from build123d import *

# Parameters (mm, degrees)
F0_R     = 6.35
F1_DEPTH = 3.81
F2_R     = 2.54
F3_DEPTH = 5.08
F6_D     = 3.175
F6_DEPTH = 2.032
F6_TIP   = 0.9538662327
F7_D     = 3.175
F7_DEPTH = 2.032
F7_TIP   = 0.9538662327


with BuildPart() as f1:
    # F0 (on Top) → F1 (new body)
    with BuildSketch(Plane.XY):
        Circle(F0_R)
    extrude(amount=F1_DEPTH)

    # F2 (on face) → F3 (join)
    with BuildSketch(Plane.XY.offset(3.81)):
        Circle(F2_R)
    extrude(amount=F3_DEPTH)

    # F6
    with Locations(Plane.XY.offset(3.81)):
        with Locations((-4.445, 0)):
            Hole(F6_D / 2, depth=F6_DEPTH)
            with Locations((0, 0, -(F6_DEPTH + F6_TIP / 2))):  # 118° drill point
                Cone(0, F6_D / 2, F6_TIP, mode=Mode.SUBTRACT)

    # F7
    with Locations(Plane.XY.offset(3.81)):
        with Locations((4.445, 0)):
            Hole(F7_D / 2, depth=F7_DEPTH)
            with Locations((0, 0, -(F7_DEPTH + F7_TIP / 2))):  # 118° drill point
                Cone(0, F7_D / 2, F7_TIP, mode=Mode.SUBTRACT)


solid = f1.part
Verification items for the finished model (mm, model axes). A direction names the side the tool comes from. Coordinates: 2 decimals unless noted, no trailing zeros. Order: outer loops, then holes, each group sorted by start corner. A loop starts at its lowest first (then second) coordinate and runs counter-clockwise, first axis right, second up.
Item 1: Section check B-B, the plane z = 4.5. Enter the section's corners in (x, y), then the cut area to 3 significant figures.
Filled in:
outline: circle Ø5.08 at (0, 0)
area: 20.3 mm2
Item 2: Release check for a two-part mould opening along Y. For faces 1 (the face through (-1.38, -6.2, 1.88)), 2 (the face through (0, 0, 0)), 3 (the face through (-4.18, 0.08, 0.99)) record: +Y half, -Y half, draft (parallel to the pull), parting line (faces both ways), or undercut.
Filled in:
face 1: parting line
face 2: draft
face 3: undercut
Item 3: Section check D-D, the plane y = -4.25. Enter the section's corners in (x, z), then the cut area to 3 significant figures.
Filled in:
outline: (-4.72, 0) - (4.72, 0) - (4.72, 3.81) - (-4.72, 3.81) - close
area: 36.0 mm2
Item 4: Access from +Z, -Z, +X, -X, +Y, -Y to the whole of each face (thin tool, end or side, straight path). Record for faces 4 (the face through (6.03, 0.07, 2.78)), 5 (the face through (0, 0, 8.89)).
Filled in:
face 4: +Z
face 5: +Z, +X, -X, +Y, -Y
Item 5: Material ranges on L1, parallel to X at y = 1, z = 3.5; L2, parallel to Z at x = -3.75, y = -1.5; L3, parallel to Y at x = 0, z = 4.75, recorded low to high.
Filled in:
L1: x = -6.27 to -5.68, -3.21 to 3.21, 5.68 to 6.27
L2: z = 0 to 3.81
L3: y = -2.54 to 2.54
Item 6: Section check A-A, the plane x = 0. Enter the section's corners in (y, z).
Filled in:
outline: (-6.35, 0) - (6.35, 0) - (6.35, 3.81) - (2.54, 3.81) - (2.54, 8.89) - (-2.54, 8.89) - (-2.54, 3.81) - (-6.35, 3.81) - close
Item 7: Depth check by flat-ended pin: pin 1 (3 mm diameter, centred on y = 2, z = 1, fed in from -X); pin 2 (1 mm diameter, centred on x = -4.5, y = -1.5, fed in from +Z); pin 3 (1 mm diameter, centred on x = 2, z = 5.5, fed in from -Y). Enter the tip coordinate at first touch or a pass-through.
Filled in:
pin 1: stops at x = -6.33
pin 2: stops at z = 3.81
pin 3: stops at y = -2.05
Item 8: Section check C-C, the plane z = 3.25. Give the number of separate pieces and of enclosed holes in the cut face, then the cut area to 3 significant figures.
Filled in:
separate pieces: 1
enclosed holes: 2
area: 111 mm2
